```python
from build123d import *

# Parameters (mm, degrees)
SKETCH1_W           = 101.6
SKETCH1_H           = 127
BOSS_EXTRUDE1_DEPTH = 6.35
SKETCH2_W           = 6.604
SKETCH2_H           = 3.302
SKETCH2_W_2         = 3.429
SKETCH2_H_2         = 6.604
CUT_EXTRUDE1_DEPTH  = 82.567226875
SKETCH3_W           = 63.5
SKETCH3_H           = 127
SKETCH3_R           = 3.429
BOSS_EXTRUDE2_DEPTH = 6.35
SKETCH4_W           = 44.45
SKETCH4_H           = 127
CUT_EXTRUDE2_DEPTH  = 131.908603613


with BuildPart() as part:
    # Sketch1 → Boss-Extrude1 (new body)
    with BuildSketch(Plane(origin=(0, 0, 0), x_dir=(1, 0, 0), z_dir=(0, 1, 0))):
        Rectangle(SKETCH1_W, SKETCH1_H)
    extrude(amount=BOSS_EXTRUDE1_DEPTH)

    # Sketch2 → Cut-Extrude1 (cut, through all)
    with BuildSketch(Plane(origin=(0, 6.35, 0), x_dir=(1, 0, 0), z_dir=(0, 1, 0))):
        with Locations((-31.75, -61.849)):
            Rectangle(SKETCH2_W, SKETCH2_H)
        with Locations((-19.05, -61.849)):
            Rectangle(SKETCH2_W, SKETCH2_H)
        with Locations((-6.35, -61.849)):
            Rectangle(SKETCH2_W, SKETCH2_H)
        with Locations((6.35, -61.849)):
            Rectangle(SKETCH2_W, SKETCH2_H)
        with Locations((19.05, -61.849)):
            Rectangle(SKETCH2_W, SKETCH2_H)
        with Locations((31.75, -61.849)):
            Rectangle(SKETCH2_W, SKETCH2_H)
        with Locations((31.75, 61.849)):
            Rectangle(SKETCH2_W, SKETCH2_H)
        with Locations((19.05, 61.849)):
            Rectangle(SKETCH2_W, SKETCH2_H)
        with Locations((6.35, 61.849)):
            Rectangle(SKETCH2_W, SKETCH2_H)
        with Locations((-6.35, 61.849)):
            Rectangle(SKETCH2_W, SKETCH2_H)
        with Locations((-19.05, 61.849)):
            Rectangle(SKETCH2_W, SKETCH2_H)
        with Locations((-31.75, 61.849)):
            Rectangle(SKETCH2_W, SKETCH2_H)
        with Locations((-49.0855, 31.75)):
            Rectangle(SKETCH2_W_2, SKETCH2_H_2)
        with Locations((-49.0855, 19.05)):
            Rectangle(SKETCH2_W_2, SKETCH2_H_2)
        with Locations((-49.0855, 6.35)):
            Rectangle(SKETCH2_W_2, SKETCH2_H_2)
        with Locations((-49.0855, -6.35)):
            Rectangle(SKETCH2_W_2, SKETCH2_H_2)
        with Locations((-49.0855, -19.05)):
            Rectangle(SKETCH2_W_2, SKETCH2_H_2)
        with Locations((-49.0855, -31.75)):
            Rectangle(SKETCH2_W_2, SKETCH2_H_2)
        with Locations((49.0855, -31.75)):
            Rectangle(SKETCH2_W_2, SKETCH2_H_2)
        with Locations((49.0855, -19.05)):
            Rectangle(SKETCH2_W_2, SKETCH2_H_2)
        with Locations((49.0855, -6.35)):
            Rectangle(SKETCH2_W_2, SKETCH2_H_2)
        with Locations((49.0855, 6.35)):
            Rectangle(SKETCH2_W_2, SKETCH2_H_2)
        with Locations((49.0855, 19.05)):
            Rectangle(SKETCH2_W_2, SKETCH2_H_2)
        with Locations((49.0855, 31.75)):
            Rectangle(SKETCH2_W_2, SKETCH2_H_2)
        with Locations((-49.0855, 44.45)):
            Rectangle(SKETCH2_W_2, SKETCH2_H_2)
        with Locations((-49.0855, -44.45)):
            Rectangle(SKETCH2_W_2, SKETCH2_H_2)
        with Locations((49.0855, -44.45)):
            Rectangle(SKETCH2_W_2, SKETCH2_H_2)
        with Locations((49.0855, 44.45)):
            Rectangle(SKETCH2_W_2, SKETCH2_H_2)
    extrude(amount=-CUT_EXTRUDE1_DEPTH, mode=Mode.SUBTRACT)

    # Sketch3 → Boss-Extrude2 (add)
    with BuildSketch(Plane(origin=(0, 6.35, 0), x_dir=(1, 0, 0), z_dir=(0, 1, 0))):
        with Locations((-82.55, 0)):
            Rectangle(SKETCH3_W, SKETCH3_H)
        with Locations(Location((-101.6, 50.8, 0), (0, 0, 270))):
            Circle(SKETCH3_R, mode=Mode.SUBTRACT)
        with Locations(Location((-88.9, 50.8, 0), (0, 0, 270))):
            Circle(SKETCH3_R, mode=Mode.SUBTRACT)
        with Locations(Location((-88.9, 38.1, 0), (0, 0, 270))):
            Circle(SKETCH3_R, mode=Mode.SUBTRACT)
        with Locations(Location((-101.6, 38.1, 0), (0, 0, 270))):
            Circle(SKETCH3_R, mode=Mode.SUBTRACT)
        with Locations(Location((-101.6, 25.4, 0), (0, 0, 270))):
            Circle(SKETCH3_R, mode=Mode.SUBTRACT)
        with Locations(Location((-88.9, 25.4, 0), (0, 0, 270))):
            Circle(SKETCH3_R, mode=Mode.SUBTRACT)
        with Locations(Location((-76.2, 50.8, 0), (0, 0, 270))):
            Circle(SKETCH3_R, mode=Mode.SUBTRACT)
        with Locations(Location((-63.5, 50.8, 0), (0, 0, 270))):
            Circle(SKETCH3_R, mode=Mode.SUBTRACT)
        with Locations(Location((-76.2, 38.1, 0), (0, 0, 270))):
            Circle(SKETCH3_R, mode=Mode.SUBTRACT)
        with Locations(Location((-63.5, 38.1, 0), (0, 0, 270))):
            Circle(SKETCH3_R, mode=Mode.SUBTRACT)
        with Locations(Location((-76.2, 25.4, 0), (0, 0, 270))):
            Circle(SKETCH3_R, mode=Mode.SUBTRACT)
        with Locations(Location((-63.5, 25.4, 0), (0, 0, 270))):
            Circle(SKETCH3_R, mode=Mode.SUBTRACT)
        with Locations(Location((-101.6, 12.7, 0), (0, 0, 270))):
            Circle(SKETCH3_R, mode=Mode.SUBTRACT)
        with Locations(Location((-88.9, 12.7, 0), (0, 0, 270))):
            Circle(SKETCH3_R, mode=Mode.SUBTRACT)
        with Locations(Location((-76.2, 12.7, 0), (0, 0, 270))):
            Circle(SKETCH3_R, mode=Mode.SUBTRACT)
        with Locations(Location((-63.5, 12.7, 0), (0, 0, 270))):
            Circle(SKETCH3_R, mode=Mode.SUBTRACT)
        with Locations(Location((-101.6, 0, 0), (0, 0, 270))):
            Circle(SKETCH3_R, mode=Mode.SUBTRACT)
        with Locations(Location((-88.9, 0, 0), (0, 0, 270))):
            Circle(SKETCH3_R, mode=Mode.SUBTRACT)
        with Locations(Location((-76.2, 0, 0), (0, 0, 270))):
            Circle(SKETCH3_R, mode=Mode.SUBTRACT)
        with Locations(Location((-63.5, 0, 0), (0, 0, 270))):
            Circle(SKETCH3_R, mode=Mode.SUBTRACT)
        with Locations(Location((-101.6, -12.7, 0), (0, 0, 270))):
            Circle(SKETCH3_R, mode=Mode.SUBTRACT)
        with Locations(Location((-88.9, -12.7, 0), (0, 0, 270))):
            Circle(SKETCH3_R, mode=Mode.SUBTRACT)
        with Locations(Location((-76.2, -12.7, 0), (0, 0, 270))):
            Circle(SKETCH3_R, mode=Mode.SUBTRACT)
        with Locations(Location((-63.5, -12.7, 0), (0, 0, 270))):
            Circle(SKETCH3_R, mode=Mode.SUBTRACT)
        with Locations(Location((-101.6, -25.4, 0), (0, 0, 270))):
            Circle(SKETCH3_R, mode=Mode.SUBTRACT)
        with Locations(Location((-88.9, -25.4, 0), (0, 0, 270))):
            Circle(SKETCH3_R, mode=Mode.SUBTRACT)
        with Locations(Location((-76.2, -25.4, 0), (0, 0, 270))):
            Circle(SKETCH3_R, mode=Mode.SUBTRACT)
        with Locations(Location((-63.5, -25.4, 0), (0, 0, 270))):
            Circle(SKETCH3_R, mode=Mode.SUBTRACT)
        with Locations(Location((-101.6, -38.1, 0), (0, 0, 270))):
            Circle(SKETCH3_R, mode=Mode.SUBTRACT)
        with Locations(Location((-88.9, -38.1, 0), (0, 0, 270))):
            Circle(SKETCH3_R, mode=Mode.SUBTRACT)
        with Locations(Location((-76.2, -38.1, 0), (0, 0, 270))):
            Circle(SKETCH3_R, mode=Mode.SUBTRACT)
        with Locations(Location((-63.5, -38.1, 0), (0, 0, 270))):
            Circle(SKETCH3_R, mode=Mode.SUBTRACT)
        with Locations(Location((-101.6, -50.8, 0), (0, 0, 270))):
            Circle(SKETCH3_R, mode=Mode.SUBTRACT)
        with Locations(Location((-88.9, -50.8, 0), (0, 0, 270))):
            Circle(SKETCH3_R, mode=Mode.SUBTRACT)
        with Locations(Location((-76.2, -50.8, 0), (0, 0, 270))):
            Circle(SKETCH3_R, mode=Mode.SUBTRACT)
        with Locations(Location((-63.5, -50.8, 0), (0, 0, 270))):
            Circle(SKETCH3_R, mode=Mode.SUBTRACT)
    extrude(amount=-BOSS_EXTRUDE2_DEPTH)

    # Sketch4 → Cut-Extrude2 (cut, through all)
    with BuildSketch(Plane(origin=(0, 6.35, 0), x_dir=(1, 0, 0), z_dir=(0, 1, 0))):
        with Locations((-92.075, 0)):
            Rectangle(SKETCH4_W, SKETCH4_H)
    extrude(amount=-CUT_EXTRUDE2_DEPTH, mode=Mode.SUBTRACT)


solid = part.part
```
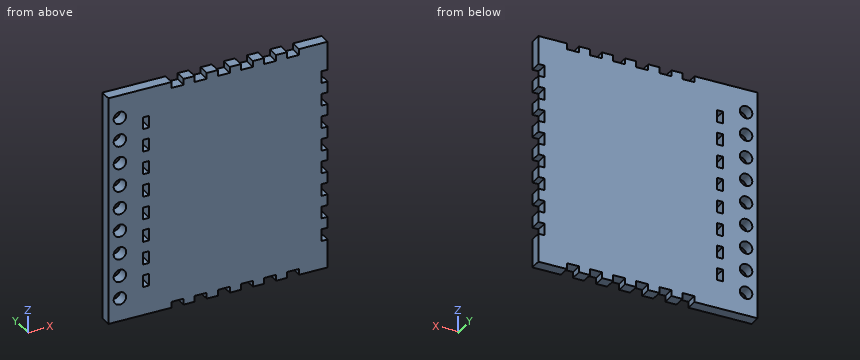
Geometry check sheet. Reference: the model listing, model coordinates, mm. Give positions to 0.01 mm unless a question says otherwise; leave off trailing zeros. Order: outer loops, then holes, each group sorted by start corner. A loop starts at its lowest first (then second) coordinate and runs counter-clockwise, first axis right, second up. Notation, with made-up numbers: (-38.75, 88.25) - (-21.75, 88.25) arc R5 cw to (-21.75, 97.25) - close; hole circle Ø1 at (85.5, -28). An arc over 180 degrees is marked (long way). Write item = value, one per line. Start each with the question number.
1) Scan lines: L1, parallel to X at y = 4, z = -50.8; L2, parallel to X at y = 2, z = 33.5; L3, parallel to Z at x = 22, y = 2. Record each from-to range of solid material in increasing order.
2) Section check A-A (z = -12.7). Enter the section's corners in (x, y).
3) Section check C-C (x = -6.5). Enter the section's corners in (y, z).
4) Gauge pin test, flat ends, axial feed: pin 1 Ø4 at (x, z) = (-63.5, 12.7) entering from -Y; pin 2 Ø1.9 at (x, y) = (6.5, 3) entering from -Z. Record the tip position at first contact, or that the pin passes through.
5) Section check B-B (y = 3.5). Count the separate pieces of the cut face and the enclosed holes in it, then the cut area to 3 significant figures.
Geometry check:
q1.L1 = -69.85 to -66.93, -60.07 to 50.8
q1.L2 = -69.85 to -50.8, -47.37 to 47.37
q1.L3 = -60.2 to 60.2
q2.outline = (-69.85, 0) - (-66.93, 0) - (-66.93, 6.35) - (-69.85, 6.35) - close; (-60.07, 0) - (50.8, 0) - (50.8, 6.35) - (-60.07, 6.35) - close
q3.outline = (0, -60.2) - (6.35, -60.2) - (6.35, 60.2) - (0, 60.2) - close
q4.pin_1 = through
q4.pin_2 = -60.2
q5.separate_pieces = 1
q5.enclosed_holes = 17
q5.area = 14,400 mm2
